```python
from build123d import *

# Parameters (mm, degrees)
F0_W     = 31.7
F0_H     = 31.7
F1_DEPTH = 19.2
F2_R     = 4.7
F2_R_2   = 3.4
F3_DEPTH = 4.6


with BuildPart() as f1:
    # F0 (on Top) → F1 (new body)
    with BuildSketch(Plane.XY):
        Rectangle(F0_W, F0_H)
    extrude(amount=F1_DEPTH)

    # F2 (on face) → F3 (join)
    with BuildSketch(Plane.XY.offset(19.2)):
        with Locations((-7.672173, 7.95)):
            Circle(F2_R)
        with Locations((-7.672173, 7.95)):
            Circle(F2_R_2, mode=Mode.SUBTRACT)
        with Locations((7.672173, 7.95)):
            Circle(F2_R)
        with Locations((7.672173, 7.95)):
            Circle(F2_R_2, mode=Mode.SUBTRACT)
        with Locations((-7.672173, -7.95)):
            Circle(F2_R)
        with Locations((-7.672173, -7.95)):
            Circle(F2_R_2, mode=Mode.SUBTRACT)
        with Locations((7.672173, -7.95)):
            Circle(F2_R)
        with Locations((7.672173, -7.95)):
            Circle(F2_R_2, mode=Mode.SUBTRACT)
    extrude(amount=F3_DEPTH)


solid = f1.part
```
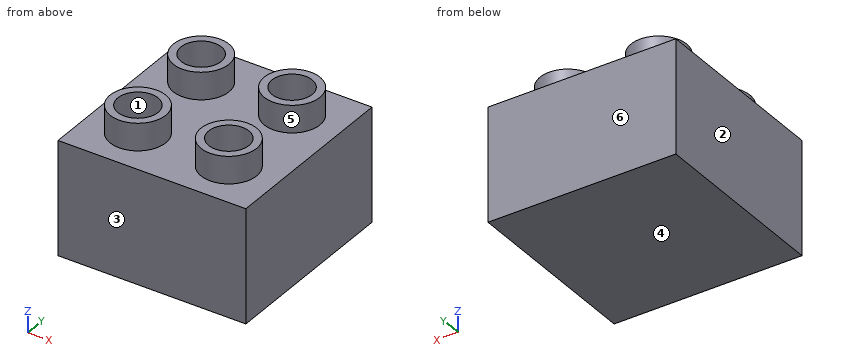
CAD build for the part. Positions are in the model's coordinates, mm. Face numbers are marked on the shaded views. A direction names the side the tool comes from. Round coordinates to 2 decimals unless told otherwise and drop trailing zeros. Write each loop counter-clockwise with the first axis right and the second up, starting at its lowest first coordinate (ties: lowest second). Pieces come first, ordered by that corner, then holes. Notation, with made-up numbers: M -37.75,-36 L -14.75,-36 A34 ccw -14.75,-4 Z; hole C 58,43.5 d2. An arc over 180 degrees is marked long. One line per question, with ' | ' between items.
1. Pin check, flat tip, straight feed: pin 1 Ø6 at (x, y) = (-7.67, -7.95) entering from +Z. Stop position of the tip, or through.
Working result:
pin 1: z = 19.2
2. Cut at D-D on y = -10. Write the cut outline in (x, z).
Working result:
outline: M -15.85,0 L 15.85,0 L 15.85,19.2 L 11.9,19.2 L 11.9,23.8 L 10.38,23.8 L 10.38,19.2 L 4.96,19.2 L 4.96,23.8 L 3.44,23.8 L 3.44,19.2 L -3.44,19.2 L -3.44,23.8 L -4.96,23.8 L -4.96,19.2 L -10.38,19.2 L -10.38,23.8 L -11.9,23.8 L -11.9,19.2 L -15.85,19.2 Z
3. Cut at B-B on y = 7.95. Write the cut outline in (x, z).
Working result:
outline: M -15.85,0 L 15.85,0 L 15.85,19.2 L 12.37,19.2 L 12.37,23.8 L 11.07,23.8 L 11.07,19.2 L 4.27,19.2 L 4.27,23.8 L 2.97,23.8 L 2.97,19.2 L -2.97,19.2 L -2.97,23.8 L -4.27,23.8 L -4.27,19.2 L -11.07,19.2 L -11.07,23.8 L -12.37,23.8 L -12.37,19.2 L -15.85,19.2 Z
4. Cut at C-C on x = -3.5. Write the cut outline in (y, z).
Working result:
outline: M -15.85,0 L 15.85,0 L 15.85,19.2 L 10.11,19.2 L 10.11,23.8 L 5.79,23.8 L 5.79,19.2 L -5.79,19.2 L -5.79,23.8 L -10.11,23.8 L -10.11,19.2 L -15.85,19.2 Z
5. Probe L1, parallel to Z at x = -12.5, y = -15; L2, parallel to Y at x = 8, z = 20. List the from-to ranges inside material, lowest first. Write a range as from..to.
Working result:
L1: 0..19.2 | L2: -12.64..-11.33, -4.57..-3.26, 3.26..4.57, 11.33..12.64
6. Mould opens along Y. For the marked faces 3, 4, 5 and 6 say: pulls with the +Y half, pulls with the -Y half, needs draft (parallel to the pull), parting line crosses it, or undercut.
Working result:
face 3: pulls with the -Y half | face 4: needs draft | face 5: undercut | face 6: pulls with the +Y half
7. Cut at A-A on z = 20.5. Write the cut outline in (x, y).
Working result:
outline: C -7.67,-7.95 d9.4; C -7.67,7.95 d9.4; C 7.67,-7.95 d9.4; C 7.67,7.95 d9.4; hole C -7.67,-7.95 d6.8; hole C -7.67,7.95 d6.8; hole C 7.67,-7.95 d6.8; hole C 7.67,7.95 d6.8
8. Which spindle directions (+Z, -Z, +X, -X, +Y, -Y) get a long thin tool onto all of the face, cutting with end or side? Do the marked faces 1 and 2. Say none if no direction does.
Working result:
face 1: +Z | face 2: +Z, -Z, -X, +Y, -Y
